from build123d import *

# Parameters (mm, degrees)
SZKIC1_W                    = 20
SZKIC1_H                    = 30
DODANIE_WYCI_GNI_CIE1_DEPTH = 40
SKORUPA3_T                  = -2
ZAOKR_GLENIE1_R             = 5
SZKIC2_W                    = 12
SZKIC2_H                    = 2
DODANIE_WYCI_GNI_CIE2_DEPTH = 2.5


with BuildPart() as part:
    # Szkic1 → Dodanie-wyciągnięcie1 (new body)
    with BuildSketch(Plane.XY):
        Rectangle(SZKIC1_W, SZKIC1_H)
    extrude(amount=DODANIE_WYCI_GNI_CIE1_DEPTH)

    # Skorupa3
    skorupa3_openings = [part.faces().sort_by_distance(p)[0] for p in [
        (0, 0, 40),
        (0, -15, 20),
    ]]
    offset(amount=SKORUPA3_T, openings=skorupa3_openings, kind=Kind.INTERSECTION)

    # Zaokrąglenie1
    zaokr_glenie1_edges = [part.edges().sort_by_distance(p)[0] for p in [
        (-10, 0, 0),
        (0, 15, 0),
        (10, 0, 0),
    ]]
    fillet(zaokr_glenie1_edges, radius=ZAOKR_GLENIE1_R)

    # Szkic2 → Dodanie-wyciągnięcie2 (add)
    with BuildSketch(Plane.XY.offset(2)):
        with Locations((0, -11)):
            Rectangle(SZKIC2_W, SZKIC2_H)
    extrude(amount=DODANIE_WYCI_GNI_CIE2_DEPTH)


solid = part.part
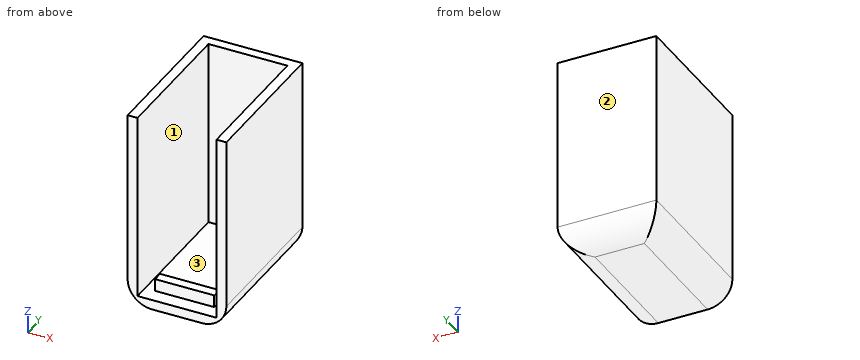
Work out the finished part from the listing and answer in its coordinate system (mm). Face numbers are marked on the shaded views. Coordinates: 2 decimals unless noted, no trailing zeros. Write each loop counter-clockwise with the first axis right and the second up, starting at its lowest first coordinate (ties: lowest second). Pieces come first, ordered by that corner, then holes. Notation, with made-up numbers: M 48,8 L 99,8 A23 cw 99,40 Z; hole C 81.5,3.5 d11. An arc over 180 degrees is marked long. Use one line per item in the form item = value. Start each with the question number.
1. The part is cut by section C-C (z = 10). Give the vertices of the cut face in (x, y), plus the area to 3 significant figures.
2. Straight lines are drawn through the part: probe 1 along X at (y, z) = (-10, 19); probe 2 along Z at (x, y) = (-2.5, -6.25); probe 3 along Y at (x, z) = (-1.25, 31.5). For each, find the intervals that lie inside material, in ascending order. Write a range as from..to.
3. The part is cut by section A-A (y = 10.5). Give the vertices of the cut face in (x, z).
4. The mould has two halves that part along Y. Classify the marked faces 1, 2 and 3: released by +Y, released by -Y, zero draft, split by the parting line, or undercut.
5. The part is cut by section D-D (x = 1.5). Give the vertices of the cut face in (y, z), plus the area to 3 significant figures.
6. The part is cut by section B-B (x = 7). Give the vertices of the cut face in (y, z).
7. Each of these flat-tipped pins is pushed along its axis until it touches: P1, Ø2, axis at x = 0.5, z = 3.5, coming from the +Y side; P2, Ø0.6, axis at y = -11, z = 3, coming from the +X side; P3, Ø1, axis at x = 5.5, z = 35.5, coming from the -Y side. Where does it stop, or does it pass through?
Evaluation:
q1.outline = M -10,-15 L -8,-15 L -8,13 L 8,13 L 8,-15 L 10,-15 L 10,15 L -10,15 Z
q1.area = 152 mm^2
q2.probe_1 = -10..-8, 8..10
q2.probe_2 = 0..2
q2.probe_3 = 13..15
q3.outline = M -10,5 A5 ccw -5.5,0.03 L 5.5,0.03 A5 ccw 10,5 L 10,40 L 8,40 L 8,2 L -8,2 L -8,40 L -10,40 Z
q4.face_1 = zero draft
q4.face_2 = released by +Y
q4.face_3 = undercut
q5.outline = M -15,0 L 10,0 A5 ccw 15,5 L 15,40 L 13,40 L 13,2 L -10,2 L -10,4.5 L -12,4.5 L -12,2 L -15,2 Z
q5.area = 136 mm^2
q6.outline = M -15,0.42 L 12,0.42 A5 ccw 15,5 L 15,40 L 13,40 L 13,2 L -15,2 Z
q7.P1 = 14.97
q7.P2 = 9.7
q7.P3 = 13
